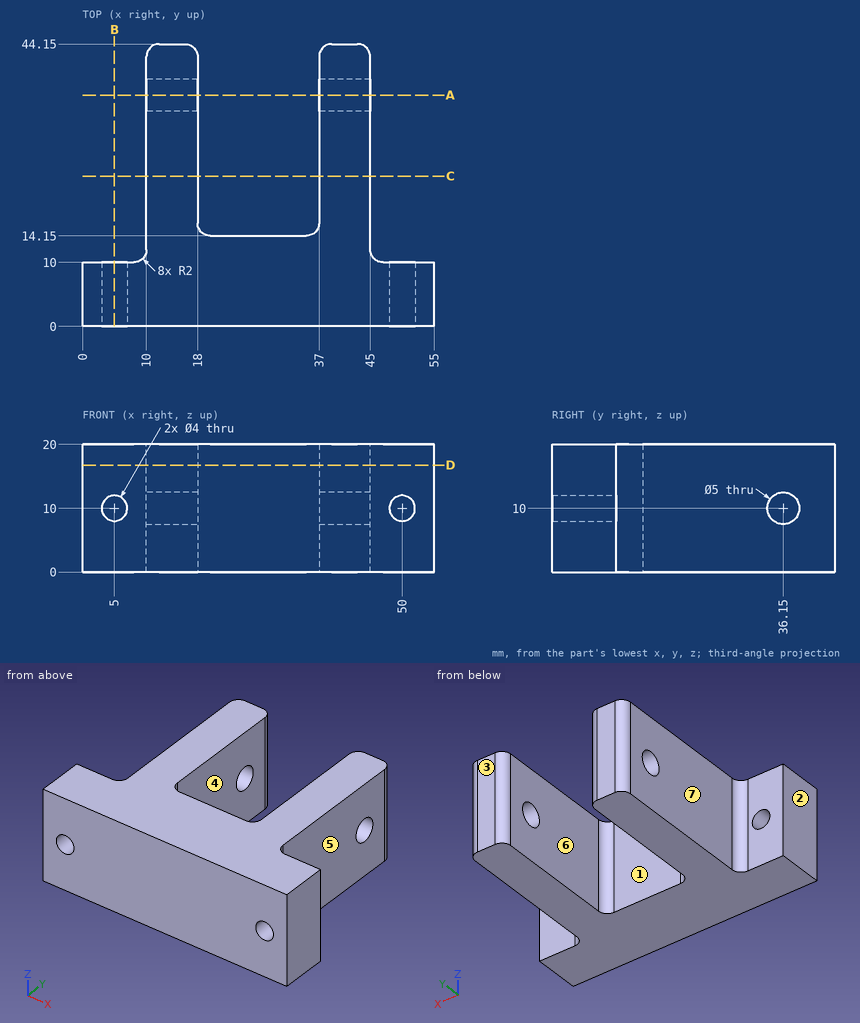
Design review of the part shown in the three views and the two pictorial views. Dimensions are in mm from the part's minimum x, y and z. A direction names the side the tool comes from. Give positions to 0.01 mm unless a question says otherwise; leave off trailing zeros. Loops run counter-clockwise (first coordinate to the right, second up) from the corner with the lowest first, then second, coordinate; pieces in that order, holes last. Notation, with made-up numbers: (19, -34.75) - (55, -34.75) arc R27 ccw to (55, -1.75) - close; hole circle Ø3 at (25.25, 87.25). An arc over 180 degrees is marked (long way). Use CSV: the item, a comma, the result in double quotes. Start each with the question number.
1. Add section C-C (y = 23.5). State the section outline as (x, z) points.
2. Machinability: for the marked faces 5, 6 and 7, which of the approach directions +Z, -Z, +X, -X, +Y, -Y give a long, thin tool a straight path to every point of the face, cutting with its end or side? Answer none if there is none.
3. Insertion check: P1, Ø7.5, axis at x = 29.5, z = 15, coming from the +Y side; P2, Ø9, axis at x = 3, z = 10.5, coming from the +Y side; P3, Ø6, axis at y = 36.15, z = 10, coming from the -X side. Each pin has a flat end and moves straight along its axis. Give the tip position at first contact, or say it passes through.
4. Add section D-D (z = 16.75). State the section outline as (x, y) points.
5. Add section A-A (y = 36.15). State the section outline as (x, z) points.
6. Add section B-B (x = 5). State the section outline as (y, z) points, plus the area to 3 significant figures.
7. Draft analysis for pull direction X (two halves, no side actions). For the marked faces 1, 2, 3 and 4, state which applies: released by +X, released by -X, zero draft, split by the parting line, or undercut.
8. Wall thickness on L1, parallel to X at y = 5.75, z = 10; L2, parallel to X at y = 35.5, z = 2.5; L3, parallel to Z at x = 5, y = 5: over which ranges is each line inside the solid? List them lowest first.
Results found:
1,outline,"(10, 0) - (18, 0) - (18, 20) - (10, 20) - close; (37, 0) - (45, 0) - (45, 20) - (37, 20) - close"
2,face 5,"+Z, -Z, +X, +Y"
2,face 6,"+Z, -Z, +Y"
2,face 7,"+Z, -Z, -X, +Y"
3,P1,"stops at y = 14.15"
3,P2,"stops at y = 10"
3,P3,"stops at x = 10"
4,outline,"(0, 0) - (55, 0) - (55, 10) - (47, 10) arc R2 cw to (45, 12) - (45, 42.15) arc R2 ccw to (43, 44.15) - (39, 44.15) arc R2 ccw to (37, 42.15) - (37, 16.15) arc R2 cw to (35, 14.15) - (20, 14.15) arc R2 cw to (18, 16.15) - (18, 42.15) arc R2 ccw to (16, 44.15) - (12, 44.15) arc R2 ccw to (10, 42.15) - (10, 12) arc R2 cw to (8, 10) - (0, 10) - close"
5,outline,"(10, 0) - (18, 0) - (18, 7.5) - (10, 7.5) - close; (10, 12.5) - (18, 12.5) - (18, 20) - (10, 20) - close; (37, 0) - (45, 0) - (45, 7.5) - (37, 7.5) - close; (37, 12.5) - (45, 12.5) - (45, 20) - (37, 20) - close"
6,outline,"(0, 0) - (10, 0) - (10, 8) - (0, 8) - close; (0, 12) - (10, 12) - (10, 20) - (0, 20) - close"
6,area,"160 mm²"
7,face 1,"undercut"
7,face 2,"released by -X"
7,face 3,"zero draft"
7,face 4,"undercut"
8,L1,"x = 0 to 3, 7 to 48, 52 to 55"
8,L2,"x = 10 to 18, 37 to 45"
8,L3,"z = 0 to 8, 12 to 20"
